from build123d import *

# Parameters (mm, degrees)
ESQUISSE1_W             = 95.41492783
ESQUISSE1_H             = 95.41492783
ESQUISSE1_R             = 3.95
ESQUISSE1_R_2           = 15
BOSS_EXTRU_1_DEPTH      = 2
BOSS_EXTRU_2_START      = 2
ESQUISSE1_3_W           = 95.41492783
ESQUISSE1_3_H           = 95.41492783
ESQUISSE1_3_R           = 15
ESQUISSE1_3_R_2         = 3.95
BOSS_EXTRU_2_DEPTH      = 10
CONG_1_R                = 7.9
CHANFREIN1_SIZE         = 2
CHANFREIN1_SIZE2        = 3.464101615
ESQUISSE4_R             = 3.15
ENL_V_MAT_EXTRU_2_DEPTH = 8


with BuildPart() as part:
    # Esquisse1 → Boss.-Extru.1 (new body)
    with BuildSketch(Plane.XY):
        Rectangle(ESQUISSE1_W, ESQUISSE1_H)
        with Locations((-40, -40)):
            Circle(ESQUISSE1_R, mode=Mode.SUBTRACT)
        with Locations((40, -40)):
            Circle(ESQUISSE1_R, mode=Mode.SUBTRACT)
        with Locations((40, 40)):
            Circle(ESQUISSE1_R, mode=Mode.SUBTRACT)
        with Locations((-40, 40)):
            Circle(ESQUISSE1_R, mode=Mode.SUBTRACT)
        Circle(ESQUISSE1_R_2, mode=Mode.SUBTRACT)
        with Locations((-40, -40)):
            Circle(ESQUISSE1_R)
        with Locations((40, -40)):
            Circle(ESQUISSE1_R)
        with Locations((40, 40)):
            Circle(ESQUISSE1_R)
        with Locations((-40, 40)):
            Circle(ESQUISSE1_R)
    extrude(amount=BOSS_EXTRU_1_DEPTH)

    # Esquisse1<3> → Boss.-Extru.2 (add)
    with BuildSketch(Plane.XY.offset(BOSS_EXTRU_2_START)):
        Rectangle(ESQUISSE1_3_W, ESQUISSE1_3_H)
        Circle(ESQUISSE1_3_R, mode=Mode.SUBTRACT)
        with Locations((-40, 40)):
            Circle(ESQUISSE1_3_R_2, mode=Mode.SUBTRACT)
        with Locations((40, 40)):
            Circle(ESQUISSE1_3_R_2, mode=Mode.SUBTRACT)
        with Locations((40, -40)):
            Circle(ESQUISSE1_3_R_2, mode=Mode.SUBTRACT)
        with Locations((-40, -40)):
            Circle(ESQUISSE1_3_R_2, mode=Mode.SUBTRACT)
    extrude(amount=BOSS_EXTRU_2_DEPTH)

    # Congé1
    cong_1_edges = [part.edges().sort_by_distance(p)[0] for p in [
        (-47.707463915, -47.707463915, 6),
        (-47.707463915, 47.707463915, 6),
        (47.707463915, 47.707463915, 6),
        (47.707463915, -47.707463915, 6),
    ]]
    fillet(cong_1_edges, radius=CONG_1_R)

    # Chanfrein1
    chanfrein1_edges = [part.edges().sort_by_distance(p)[0] for p in [
        (0, 47.707463915, 12),
        (47.707463915, 0, 12),
        (-47.707463915, 0, 12),
        (0, -47.707463915, 12),
        (-45.393607486, 45.393607486, 12),
        (-45.393607486, -45.393607486, 12),
        (45.393607486, -45.393607486, 12),
        (45.393607486, 45.393607486, 12),
    ]]
    chanfrein1_side = [part.faces().sort_by_distance(p)[0] for p in [
        (0, -46.358093065, 12),
    ]]
    chamfer(chanfrein1_edges, length=CHANFREIN1_SIZE, length2=CHANFREIN1_SIZE2, reference=chanfrein1_side[0])

    # Esquisse4 → Enlèv. mat.-Extru.2 (cut)
    with BuildSketch(Plane(origin=(0, 0, 0), x_dir=(-1, 0, 0), z_dir=(0, 0, -1))):
        with Locations((-30, 30)):
            Circle(ESQUISSE4_R)
        with Locations((-30, -30)):
            Circle(ESQUISSE4_R)
        with Locations((30, -30)):
            Circle(ESQUISSE4_R)
        with Locations((30, 30)):
            Circle(ESQUISSE4_R)
    extrude(amount=-ENL_V_MAT_EXTRU_2_DEPTH, mode=Mode.SUBTRACT)


solid = part.part
Design review of the part built by this model. Coordinates are the model's own, in mm. A direction names the side the tool comes from. Round coordinates to 2 decimals unless told otherwise and drop trailing zeros. Order: outer loops, then holes, each group sorted by start corner. A loop starts at its lowest first (then second) coordinate and runs counter-clockwise, first axis right, second up. Notation, with made-up numbers: M 63.5,-39.5 L 98.5,-39.5 A11 ccw 98.5,-23.5 Z; hole C 81,14.25 d5. An arc over 180 degrees is marked long. Answer as CSV lines item,"result". Start each with the question number.
1) Tool access review of faces 5 (the face through (-37.877, 43.331, 6.93)), 6 (the face through (-30, 30, 8)), 7 (the face through (-47.707, -1, 4)): name each direction out of +Z, -Z, +X, -X, +Y, -Y from which nothing blocks a thin tool from reaching the whole face with its end or side.
2) Add section C-C (x = 12). Give the boundary of the cut face in (y, z).
3) Add section B-B (z = 3.5). Give the number of separate pieces and of enclosed holes in the cut face, then the cut area to 3 significant figures.
4) Add section D-D (y = 30). Give the boundary of the cut face in (x, z), then the cut area to 3 significant figures.
5) Wall thickness on line 1 along Y through (x, z) = (40, 6.75); line 2 along X through (y, z) = (-30.5, 3.75); line 3 along Y through (x, z) = (0, 3.5): over which ranges is each line inside the solid? List them lowest first. Write a range as [from, to].
6) Add section A-A (y = 0). Give the boundary of the cut face in (x, z).
7) For pin 1 Ø2.5 at (x, y) = (38.5, 41) entering from +Z; pin 2 Ø3 at (x, y) = (30, -29.5) entering from -Z, all flat-tipped, find the tip position at first contact; note any pin that passes through.
8) The part is to be moulded in two halves that separate along X. For faces 1 (the face through (0.557, -46.721, 10.244)), 2 (the face through (27.09, 28.79, 3.94)), 3 (the face through (46.721, 0.557, 10.244)), 4 (the face through (-46.721, -0.557, 10.244)), say which applies: +X half, -X half, draft (parallel to the pull), parting line (faces both ways), or undercut.
Resolved:
1,face 5,"+Z"
1,face 6,"-Z"
1,face 7,"+Z, -Z, -X, +Y, -Y"
2,outline,"M -47.71,0 L -9,0 L -9,12 L -45.71,12 L -47.71,8.54 Z; M 9,0 L 47.71,0 L 47.71,8.54 L 45.71,12 L 9,12 Z"
3,separate pieces,"1"
3,enclosed holes,"9"
3,area,"8,020 mm^2"
4,outline,"M -47.71,0 L -33.15,0 L -33.15,8 L -26.85,8 L -26.85,0 L 26.85,0 L 26.85,8 L 33.15,8 L 33.15,0 L 47.71,0 L 47.71,8.54 L 45.71,12 L -45.71,12 L -47.71,8.54 Z"
4,area,"1,040 mm^2"
5,line 1,"[-47.71, -43.95], [-36.05, 36.05], [43.95, 47.71]"
5,line 2,"[-47.71, -33.11], [-26.89, 26.89], [33.11, 47.71]"
5,line 3,"[-47.71, -15], [15, 47.71]"
6,outline,"M -47.71,0 L -15,0 L -15,12 L -45.71,12 L -47.71,8.54 Z; M 15,0 L 47.71,0 L 47.71,8.54 L 45.71,12 L 15,12 Z"
7,pin 1,"z = 2"
7,pin 2,"z = 8"
8,face 1,"draft"
8,face 2,"undercut"
8,face 3,"+X half"
8,face 4,"-X half"
